Build history of the part. All positions in model axes, mm. A direction names the side the tool comes from. Round coordinates to 2 decimals unless told otherwise and drop trailing zeros. Write each loop counter-clockwise with the first axis right and the second up, starting at its lowest first coordinate (ties: lowest second). Pieces come first, ordered by that corner, then holes. Notation, with made-up numbers: (49, -36.5) - (74, -36.5) arc R6 ccw to (74, -30.5) - close; hole circle Ø11 at (43, -29.75). An arc over 180 degrees is marked (long way). Write each question's results on one line, items separated by ' | '.
from build123d import *

# Parameters (mm, degrees)
F0_W          = 40
F0_H          = 40
F1_DEPTH      = 3
F2_R          = 2
F3_DEPTH      = 25
F5_DEPTH      = 30
F7_DEPTH      = 36.001
F9_DEPTH      = 36.001
F11_DEPTH     = 36.001
F12_T         = 2.5
F12_T3_DEPTH  = 21.4924225025
F12_T5_DEPTH  = 21.4924225025
F12_T8_ANGLE  = 35.4679110995
F12_T10_ANGLE = 35.4679110995
F12_T12_ANGLE = 35.4679110995
F12_T14_ANGLE = 35.4679110995
F13_W         = 30
F13_H         = 5.7462014769
F14_DEPTH     = 25


# Not quite as in the source:
# - a shell that OpenCascade refuses in one call is made with other operations: the cavity is built on its own and cut out


with BuildPart() as f1:
    # F0 (on Top) → F1 (new body)
    with BuildSketch(Plane.XY):
        with Locations((20, 20)):
            Rectangle(F0_W, F0_H)
    extrude(amount=F1_DEPTH)

    # F2 (on face) → F3 (cut)
    with BuildSketch(Plane.XY.offset(3)):
        with Locations((4, 36)):
            Circle(F2_R)
        with Locations((36, 36)):
            Circle(F2_R)
        with Locations((36, 4)):
            Circle(F2_R)
        with Locations((4, 4)):
            Circle(F2_R)
    extrude(amount=-F3_DEPTH, mode=Mode.SUBTRACT)

    # F4 (on face) → F5 (join)
    with BuildSketch(Plane.XY.offset(3)):
        with BuildLine():
            Line((28.2462112512, 36), (11.7537887488, 36))
            ThreePointArc((11.7537887488, 36), (7.2720779386, 32.7279220614), (4, 28.2462112512))
            Line((4, 28.2462112512), (4, 11.7537887488))
            ThreePointArc((4, 11.7537887488), (7.2720779386, 7.2720779386), (11.7537887488, 4))
            Line((11.7537887488, 4), (28.2462112512, 4))
            ThreePointArc((28.2462112512, 4), (32.7279220614, 7.2720779386), (36, 11.7537887488))
            Line((36, 11.7537887488), (36, 28.2462112512))
            ThreePointArc((36, 28.2462112512), (32.7279220614, 32.7279220614), (28.2462112512, 36))
        make_face()
    extrude(amount=F5_DEPTH)

    # F6 (on face) → F7 (cut, through all)
    with BuildSketch(Plane.YZ.offset(36)):
        Polygon((2.4936108384, 3), (39.5666994154, 38.5907627642), (48.4694316983, 41.8781600893), (2.4936108384, 41.8781600893), align=None)
    extrude(amount=-F7_DEPTH, mode=Mode.SUBTRACT)

    # F8 (on face) → F9 (cut, through all)
    with BuildSketch(Plane.YZ.offset(36)):
        Polygon((20.7161400467, 23.8601379097), (36.8017591536, 4.2844121344), (40.8149436116, 38.1976142526), (20.7161400467, 38.1976142526), align=None)
    extrude(amount=-F9_DEPTH, mode=Mode.SUBTRACT)

    # F10 (on face) → F11 (cut, through all)
    with BuildSketch(Plane.YZ.offset(36)):
        Polygon((13.3647378534, 17.821257934), (36.5101168772, 17.821257934), (38.6116616428, 31.5769352019), (13.3647378534, 31.5769352019), align=None)
    extrude(amount=-F11_DEPTH, mode=Mode.SUBTRACT)

    # F12: shell of thickness 2.5, made by hand


with BuildPart() as f12_core1:
    # F12_t2: copy of F1
    add(f1.part)

    # the walls: a layer under each face that stays
    f12_faces = [f12_core1.faces().sort_by_distance(p)[0] for p in [
        (0, 20, 1.5),
        (20, 40, 1.5),
        (20, 0, 1.5),
        (6.6666666667, 6.6666666667, 3),
        (40, 20, 1.5),
        (2, 4, 1.5),
        (34, 4, 1.5),
        (2, 36, 1.5),
        (34, 36, 1.5),
        (36, 20, 10.410628967),
        (32.7279220614, 7.2720779386, 7.444960048),
        (32.7279220614, 32.7279220614, 8.8481312629),
        (20, 4, 3.7230789413),
        (20, 36, 4.1300647323),
        (7.2720779386, 7.2720779386, 7.444960048),
        (7.2720779386, 32.7279220614, 8.8481312629),
        (4, 20, 10.410628967),
        (20, 30.8391816878, 11.5406936993),
        (20, 21.8052626371, 17.821257934),
        (20, 10.9660809493, 11.1337079083),
    ]]
    thicken(f12_faces, amount=-F12_T, mode=Mode.SUBTRACT)

    # F12_s4 → F12_t3 (cut)
    with BuildSketch(Plane.XZ.offset(-30.7462112512)):
        Polygon((36.025, 3.025), (36, 0.5), (33.5, 0.5), (33.5, 3), align=None)
        Polygon((3.975, 3.025), (4, 0.5), (6.5, 0.5), (6.5, 3), align=None)
    extrude(amount=F12_T3_DEPTH, mode=Mode.SUBTRACT)

    # F12_s6 → F12_t5 (cut)
    with BuildSketch(Plane.YZ.offset(9.2537887488)):
        Polygon((3.975, 3.025), (4, 0.5), (6.5, 0.5), (6.5, 3), align=None)
        Polygon((36.025, 3.025), (36, 0.5), (33.5, 0.5), (33.5, 3), align=None)
    extrude(amount=F12_T5_DEPTH, mode=Mode.SUBTRACT)

    # F12_s7 → F12_t8 (revolve, cut)
    with BuildSketch(Plane(origin=(23.9468753099, 12.3419370383, 0), x_dir=(0, 0, 1), z_dir=(-0.8888888889, -0.4581228473, 0))):
        Polygon((3.025, -9.409679168), (0.5, -9.384679168), (0.5, -6.884679168), (3, -6.884679168), align=None)
    revolve(axis=Axis((20, 20, 3), (0, 0, 1)), revolution_arc=F12_T8_ANGLE, mode=Mode.SUBTRACT)

    # F12_s9 → F12_t10 (revolve, cut)
    with BuildSketch(Plane(origin=(-3.9468753099, 7.6580629617, 0), x_dir=(0, 0, 1), z_dir=(0.4581228473, -0.8888888889, 0))):
        Polygon((3.025, -44.9652347236), (0.5, -44.9402347236), (0.5, -42.4402347236), (3, -42.4402347236), align=None)
    revolve(axis=Axis((20, 20, 3), (0, 0, 1)), revolution_arc=F12_T10_ANGLE, mode=Mode.SUBTRACT)

    # F12_s11 → F12_t12 (revolve, cut)
    with BuildSketch(Plane(origin=(-3.9468753099, 7.6580629617, 0), x_dir=(0, 0, 1), z_dir=(-0.4581228473, 0.8888888889, 0))):
        Polygon((3.025, 8.9152347236), (0.5, 8.9402347236), (0.5, 11.4402347236), (3, 11.4402347236), align=None)
    revolve(axis=Axis((20, 20, 3), (0, 0, 1)), revolution_arc=F12_T12_ANGLE, mode=Mode.SUBTRACT)

    # F12_s13 → F12_t14 (revolve, cut)
    with BuildSketch(Plane(origin=(23.9468753099, 12.3419370383, 0), x_dir=(0, 0, 1), z_dir=(0.8888888889, 0.4581228473, 0))):
        Polygon((3.025, -26.640320832), (0.5, -26.615320832), (0.5, -24.115320832), (3, -24.115320832), align=None)
    revolve(axis=Axis((20, 20, 3), (0, 0, 1)), revolution_arc=F12_T14_ANGLE, mode=Mode.SUBTRACT)


with BuildPart() as f1_1:
    add(f1.part)

    # what is left inside the walls is the cavity
    f12_cavity = [f12_core1.part.solids().sort_by_distance(p)[0] for p in [
        (20, 14.166667, 0.025),
    ]]
    add(f12_cavity, mode=Mode.SUBTRACT)

    # F13 (on face) → F14 (cut)
    with BuildSketch(Plane.XY.offset(17.821257934)):
        with Locations((20, 21.8052626371)):
            Rectangle(F13_W, F13_H)
    extrude(amount=-F14_DEPTH, mode=Mode.SUBTRACT)


solid = f1_1.part
(1) Two-plate mould, pull along X, no slides. Class faces 5 (the flat face through (33.5, 16, 6)), 6 (the flat face through (20.22, 10.87, 11.04)), 7 (the cylindrical face through (33.624, 31.764, 7.467)), 8 (the flat face through (6.5, 26, 6)): released by +X, released by -X, zero draft, split by the parting line, or undercut.
Worked answers:
face 5: undercut | face 6: zero draft | face 7: released by +X | face 8: undercut
(2) Tool access for faces 1 (the flat face through (20, 33.5, 2)), 2 (the cylindrical face through (6.376, 8.236, 6.395)), 3 (the flat face through (35, 22, 9)), 4 (the flat face through (0, 20, 1)): list every direction of +Z, -Z, +X, -X, +Y, -Y with a clear straight run to the whole face (end or side of a thin tool).
Worked answers:
face 1: -Z | face 2: +Z, -X, -Y | face 3: +Z, -Z | face 4: +Z, -Z, -X, +Y, -Y
(3) Slice it at B-B, the plane x = 5.5. Write the cut outline in (y, z).
Worked answers:
outline: (0, 0) - (2.68, 0) - (2.68, 3) - (0, 3) - close; (5.32, 0) - (8.24, 0) - (8.24, 0.5) - (18.93, 0.5) - (18.93, 17.82) - (17.93, 17.82) - (9.33, 9.57) - (9.33, 3) - (5.32, 3) - close; (24.68, 0.5) - (31.76, 0.5) - (31.76, 0) - (34.68, 0) - (34.68, 3) - (30.67, 3) - (30.67, 11.75) - (25.68, 17.82) - (24.68, 17.82) - close; (37.32, 0) - (40, 0) - (40, 3) - (37.32, 3) - close
(4) Drill centre lines: probe 1 along X at (y, z) = (4, 1.2); probe 2 along X at (y, z) = (25.5, 4.25). Where is each one in solid material? Low to high. Write a range as [from, to].
Worked answers:
probe 1: x = [0, 2], [6, 34], [38, 40] | probe 2: x = [4, 6.5], [33.5, 36]
(5) Slice it at C-C, the plane x = 37. Write the cut outline in (y, z).
Worked answers:
outline: (0, 0) - (2.27, 0) - (2.27, 3) - (0, 3) - close; (5.73, 0) - (8.39, 0) - (8.39, 0.5) - (31.61, 0.5) - (31.61, 0) - (34.27, 0) - (34.27, 3) - (5.73, 3) - close; (37.73, 0) - (40, 0) - (40, 3) - (37.73, 3) - close
(6) Slice it at D-D, the plane y = 16.5. Write the cut outline in (x, z), and give its area (3 significant figures).
Worked answers:
outline: (0, 0) - (2.5, 0) - (2.5, 0.5) - (6.5, 0.5) - (6.5, 12.98) - (33.5, 12.98) - (33.5, 0.5) - (37.5, 0.5) - (37.5, 0) - (40, 0) - (40, 3) - (36, 3) - (36, 16.45) - (4, 16.45) - (4, 3) - (0, 3) - close | area: 196 mm2
(7) Slice it at A-A, the plane z = 1.5. Write the cut outline in (x, y), and give its area (3 significant figures).
Worked answers:
outline: (0, 0) - (40, 0) - (40, 40) - (0, 40) - close; hole circle Ø4 at (4, 4); hole circle Ø4 at (4, 36); hole (5, 18.93) - (6.5, 18.93) - (6.5, 12.38) arc R15.5 ccw to (12.38, 6.5) - (27.62, 6.5) arc R15.5 ccw to (33.5, 12.38) - (33.5, 18.93) - (35, 18.93) - (35, 24.68) - (33.5, 24.68) - (33.5, 27.62) arc R15.5 ccw to (27.62, 33.5) - (12.38, 33.5) arc R15.5 ccw to (6.5, 27.62) - (6.5, 24.68) - (5, 24.68) - close; hole circle Ø4 at (36, 4); hole circle Ø4 at (36, 36) | area: 860 mm2
(8) Flat gauge pins, fed straight in: pin 1 Ø2 at (x, z) = (9, 10.5) entering from -Y; pin 2 Ø7 at (y, z) = (14.5, 11) entering from +X; pin 3 Ø6 at (y, z) = (29, 13) entering from -X; pin 4 Ø2.5 at (x, y) = (36, 4) entering from -Z. Where does each tip first touch, or does it go through?
Worked answers:
pin 1: stops at y = 9.26 | pin 2: stops at x = 36 | pin 3: stops at x = 4 | pin 4: passes through
